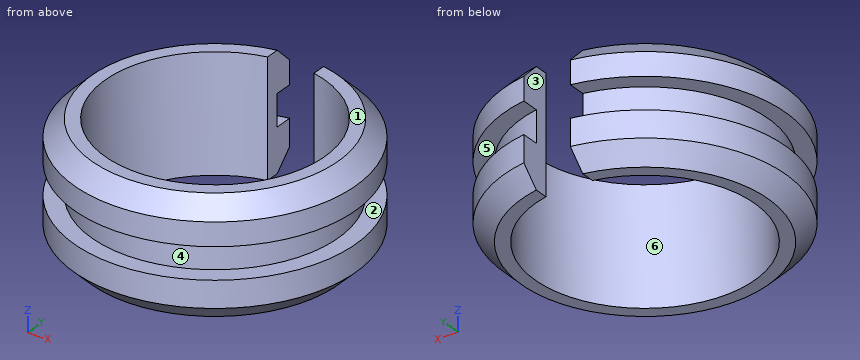
```python
from build123d import *

# Parameters (mm, degrees)
F1_DEPTH = 12.7
F2_W     = 2.116344
F2_H     = 3.450806
F4_SIZE  = 1.905


with BuildPart() as f1:
    # F0 (on Top) → F1 (new body)
    with BuildSketch(Plane.XY):
        with BuildLine():
            ThreePointArc((2.54, 11.729638), (0, -12.0015), (-2.54, 11.729638))
            Line((-2.54, 11.729638), (-2.54, 15.155629))
            ThreePointArc((-2.54, 15.155629), (0, -15.367), (2.54, 15.155629))
            Line((2.54, 15.155629), (2.54, 11.729638))
        make_face()
    extrude(amount=F1_DEPTH)

    # F2 (on Front) → F3 (revolve, cut)
    with BuildSketch(Plane.XZ):
        with Locations((14.520172, 6.529597)):
            Rectangle(F2_W, F2_H)
    revolve(axis=Axis((0, 0, 7.00403), (0, 0, -1)), mode=Mode.SUBTRACT)

    # F4
    f4_edges = [f1.edges().sort_by_distance(p)[0] for p in [
        (0, -15.367, 12.7),
        (0, -15.367, 0),
    ]]
    chamfer(f4_edges, length=F4_SIZE)


solid = f1.part
```
Source: CAD feature listing. Evaluate the final solid. Frame: model axes, mm. Face numbers are marked on the shaded views. A direction names the side the tool comes from. Give positions to 0.01 mm unless a question says otherwise; leave off trailing zeros. Write each loop counter-clockwise with the first axis right and the second up, starting at its lowest first coordinate (ties: lowest second). Pieces come first, ordered by that corner, then holes. Notation, with made-up numbers: (70, -0.75) - (87, -0.75) arc R31 cw to (87, 23.25) - close; hole circle Ø6 at (85, 73). An arc over 180 degrees is marked (long way). One line per item, written item: value. Start each with the question number.
Q1. Section query B-B, the plane x = 0. Return the cut outline in (y, z) (1 decimal), then the cut area to 3 significant figures.
Q2. Material intervals for probe 1 along X at (y, z) = (0, 4.5); probe 2 along X at (y, z) = (0, 5.75); probe 3 along Z at (x, y) = (12.5, 5.5) (1 decimal), sorted ascending. Write a range as from..to.
Q3. Set-up query: the marked faces 1, 2 and 3. Return all of +Z, -Z, +X, -X, +Y, -Y with unobstructed straight access to the full face (end or side cutting, diameter ignored); none if empty.
Q4. First-contact query: pin 1 Ø4 at (x, z) = (7.5, 11) entering from -Y (3 decimals); pin 2 Ø5 at (y, z) = (8, 11.5) entering from +X; pin 3 Ø6 at (x, z) = (12, 2.5) entering from -Y. Flat tips, straight axial feed; report the tip coordinate or a pass-through.
Q5. Section query C-C, the plane z = 9.5. Return the cut outline in (x, y), then the cut area to 3 significant figures.
Q6. Section query A-A, the plane y = 0. Return the cut outline in (x, z) (1 decimal), then the cut area to 3 significant figures.
Q7. Draft query along X for the marked faces 4, 5 and 6. Return one class per face: +X half, -X half, draft (parallel to the pull), parting line (faces both ways), or undercut.
Q8. Section query D-D, the plane z = 11.5. Return the cut outline in (x, y).
Answer:
1. outline: (-15.4, 1.9) - (-13.5, 0) - (-12, 0) - (-12, 12.7) - (-13.5, 12.7) - (-15.4, 10.8) - (-15.4, 8.3) - (-13.5, 8.3) - (-13.5, 4.8) - (-15.4, 4.8) - close
1. area: 32.5 mm2
2. probe 1: x = -15.37..-12, 12..15.37
2. probe 2: x = -13.46..-12, 12..13.46
2. probe 3: z = 0.2..4.8, 8.3..12.5
3. face 1: +Z, +X, -X, +Y, -Y
3. face 2: none
3. face 3: +Z, -Z, +Y
4. pin 1: stops at y = -14.345
4. pin 2: stops at x = 14.31
4. pin 3: stops at y = -12.46
5. outline: (-2.54, 11.73) - (-2.54, 15.16) arc R15.37 ccw (long way) to (2.54, 15.16) - (2.54, 11.73) arc R12 cw (long way) to start
5. area: 272 mm2
6. outline: (-15.4, 1.9) - (-13.5, 0) - (-12, 0) - (-12, 12.7) - (-13.5, 12.7) - (-15.4, 10.8) - (-15.4, 8.3) - (-13.5, 8.3) - (-13.5, 4.8) - (-15.4, 4.8) - close; (12, 0) - (13.5, 0) - (15.4, 1.9) - (15.4, 4.8) - (13.5, 4.8) - (13.5, 8.3) - (15.4, 8.3) - (15.4, 10.8) - (13.5, 12.7) - (12, 12.7) - close
6. area: 65.1 mm2
7. face 4: parting line
7. face 5: draft
7. face 6: undercut
8. outline: (-2.54, 11.73) - (-2.54, 14.44) arc R14.66 ccw (long way) to (2.54, 14.44) - (2.54, 11.73) arc R12 cw (long way) to start
